from build123d import *

# Parameters (mm, degrees)
SKETCH2_W           = 100
SKETCH2_H           = 100
BOSS_EXTRUDE1_DEPTH = 100
SKETCH3_R           = 5
BOSS_EXTRUDE2_DEPTH = 60
FILLET5_R           = 10


with BuildPart() as part:
    # Sketch2 → Boss-Extrude1 (new body)
    with BuildSketch(Plane(origin=(0, 0, 0), x_dir=(1, 0, 0), z_dir=(0, 1, 0))):
        with Locations((50, 50)):
            Rectangle(SKETCH2_W, SKETCH2_H)
    extrude(amount=BOSS_EXTRUDE1_DEPTH)

    # Sketch3 → Boss-Extrude2 (add)
    with BuildSketch(Plane(origin=(100, 0, 0), x_dir=(0, 0, -1), z_dir=(1, 0, 0))):
        with Locations((50, 50)):
            Circle(SKETCH3_R)
    extrude(amount=BOSS_EXTRUDE2_DEPTH)

    # Fillet5
    fillet5_edges = [part.edges().sort_by_distance(p)[0] for p in [
        (100, 100, -50),
        (50, 100, -100),
        (100, 50, -45),
        (0, 100, -50),
        (50, 0, -100),
        (100, 0, -50),
        (50, 0, 0),
        (0, 0, -50),
        (50, 100, 0),
        (0, 50, -100),
        (100, 50, -100),
        (100, 50, 0),
        (0, 50, 0),
    ]]
    fillet(fillet5_edges, radius=FILLET5_R)


solid = part.part
Can you work these out from the model? Positions are in its coordinate system, mm. A direction names the side the tool comes from. Coordinates: 2 decimals unless noted, no trailing zeros. Loops run counter-clockwise (first coordinate to the right, second up) from the corner with the lowest first, then second, coordinate; pieces in that order, holes last. Notation, with made-up numbers: (8.25, -31) - (42.25, -31) arc R25 cw to (42.25, 7) - close; hole circle Ø2 at (-7, -19.5). An arc over 180 degrees is marked (long way). Put each result on its own line as item: value. Start each with the question number.
Item 1: Suppose I cut it at C-C (x = 124). Please give me the cut outline in (y, z).
Item 2: Suppose I cut it at D-D (z = -86). Please give me the cut outline in (x, y), and give its area (3 significant figures).
Item 3: For pin 1 (3 mm diameter, centred on y = 30.5, z = -47, fed in from +X); pin 2 (3 mm diameter, centred on x = 95.5, y = 57, fed in from +Z); pin 3 (12 mm diameter, centred on x = 99, z = -19.5, fed in from -Y), each with a flat end and sliding along its axis, tell me the tip position at first contact or that it passes through.
Item 4: If I drill on line 1 along X through (y, z) = (36.5, -35); line 2 along X through (y, z) = (40, -47); line 3 along Y through (x, z) = (73, -4.5), over which ranges is the centre line in solid material (lowest first)?
Item 5: Suppose I cut it at B-B (y = 77). Please give me the cut outline in (x, z), and give its area (3 significant figures).
Item 6: Which directions (+Z, -Z, +X, -X, +Y, -Y) give clear straight access to the entire face, cutting with the end or side of a thin tool? Please do faces 1 (the face through (134.65, 54.957, -49.349)), 2 (the face through (160, 50, -50)).
Item 7: Suppose I cut it at A-A (z = -50). Please give me the cut outline in (x, y), and give its area (3 significant figures).
Here are the results:
1. outline: circle Ø10 at (50, -50)
2. outline: (0, 10) arc R10 ccw to (10, 0) - (90, 0) arc R10 ccw to (100, 10) - (100, 90) arc R10 ccw to (90, 100) - (10, 100) arc R10 ccw to (0, 90) - close
2. area: 9,910 mm²
3. pin 1: x = 100
3. pin 2: z = -0.83
3. pin 3: y = 0.46
4. line 1: 0 to 100
4. line 2: 0 to 101.1
4. line 3: 1.65 to 98.35
5. outline: (0, -90) arc R10 ccw to (10, -100) - (90, -100) arc R10 ccw to (100, -90) - (100, -10) arc R10 ccw to (90, 0) - (10, 0) arc R10 ccw to (0, -10) - close
5. area: 9,910 mm²
6. face 1: +X
6. face 2: +Z, -Z, +X, +Y, -Y
7. outline: (0, 10) arc R10 ccw to (10, 0) - (90, 0) arc R10 ccw to (100, 10) - (100, 35) arc R10 cw to (110, 45) - (160, 45) - (160, 55) - (110, 55) arc R10 cw to (100, 65) - (100, 90) arc R10 ccw to (90, 100) - (10, 100) arc R10 ccw to (0, 90) - close
7. area: 10,600 mm²
